```python
from build123d import *

# Parameters (mm, degrees)
ESQUISSE1_W             = 70
ESQUISSE1_H             = 55
ESQUISSE1_W_2           = 10
BOSS_EXTRU_1_DEPTH      = 2
ESQUISSE2_R             = 3.5
BOSS_EXTRU_2_DEPTH      = 6
ESQUISSE3_R             = 1.45
ENL_V_MAT_EXTRU_1_DEPTH = 4
ESQUISSE9_W             = 10
ESQUISSE9_H             = 55
BOSS_EXTRU_3_DEPTH      = 2
ESQUISSE10_R            = 6
ENL_V_MAT_EXTRU_8_DEPTH = 2
CONG_2_R                = 5
BOSS_EXTRU_4_DEPTH      = 5
BOSS_EXTRU_5_DEPTH      = 2
ESQUISSE15_R            = 2.15
BOSS_EXTRU_7_DEPTH      = 5
ESQUISSE17_W            = 8
ESQUISSE17_H            = 3
ENL_V_MAT_EXTRU_9_DEPTH = 10
CONG_3_R                = 1


with BuildPart() as part:
    # Esquisse1 → Boss.-Extru.1 (new body)
    with BuildSketch(Plane(origin=(0, 0, 0), x_dir=(1, 0, 0), z_dir=(0, 1, 0))):
        Rectangle(ESQUISSE1_W, ESQUISSE1_H)
        with Locations((-40, 0)):
            Rectangle(ESQUISSE1_W_2, ESQUISSE1_H)
    extrude(amount=BOSS_EXTRU_1_DEPTH)

    # Esquisse2 → Boss.-Extru.2 (add)
    with BuildSketch(Plane(origin=(0, 2, 0), x_dir=(1, 0, 0), z_dir=(0, 1, 0))):
        with Locations(Location((-11, 17.5, 0), (0, 0, 270))):
            Circle(ESQUISSE2_R)
        with Locations(Location((24, 17.5, 0), (0, 0, 270))):
            Circle(ESQUISSE2_R)
        with Locations(Location((24, -17.5, 0), (0, 0, 270))):
            Circle(ESQUISSE2_R)
        with Locations(Location((-11, -17.5, 0), (0, 0, 270))):
            Circle(ESQUISSE2_R)
    extrude(amount=BOSS_EXTRU_2_DEPTH)

    # Esquisse3 → Enlèv. mat.-Extru.1 (cut)
    with BuildSketch(Plane(origin=(0, 8, 0), x_dir=(1, 0, 0), z_dir=(0, 1, 0))):
        with Locations(Location((-11, 17.5, 0), (0, 0, 270))):
            Circle(ESQUISSE3_R)
        with Locations(Location((24, 17.5, 0), (0, 0, 270))):
            Circle(ESQUISSE3_R)
        with Locations(Location((24, -17.5, 0), (0, 0, 270))):
            Circle(ESQUISSE3_R)
        with Locations(Location((-11, -17.5, 0), (0, 0, 270))):
            Circle(ESQUISSE3_R)
    extrude(amount=-ENL_V_MAT_EXTRU_1_DEPTH, mode=Mode.SUBTRACT)

    # Esquisse9 → Boss.-Extru.3 (add)
    with BuildSketch(Plane(origin=(0, 2, 0), x_dir=(1, 0, 0), z_dir=(0, 1, 0))):
        with Locations((40, 0)):
            Rectangle(ESQUISSE9_W, ESQUISSE9_H)
    extrude(amount=-BOSS_EXTRU_3_DEPTH)

    # Esquisse10 → Enlèv. mat.-Extru.8 (cut)
    with BuildSketch(Plane(origin=(0, 2, 0), x_dir=(1, 0, 0), z_dir=(0, 1, 0))):
        with Locations(Location((35, 0, 0), (0, 0, 270))):
            Circle(ESQUISSE10_R)
    extrude(amount=-ENL_V_MAT_EXTRU_8_DEPTH, mode=Mode.SUBTRACT)

    # Congé2
    cong_2_edges = [part.edges().sort_by_distance(p)[0] for p in [
        (45, 1, -27.5),
        (45, 1, 27.5),
        (-45, 1, 27.5),
        (-45, 1, -27.5),
    ]]
    fillet(cong_2_edges, radius=CONG_2_R)

    # Esquisse12 → Boss.-Extru.4 (add)
    with BuildSketch(Plane(origin=(0, 2, 0), x_dir=(1, 0, 0), z_dir=(0, 1, 0))):
        with BuildLine():
            Line((40, 27.5), (-40, 27.5))
            ThreePointArc((-40, 27.5), (-43.535533906, 26.035533906), (-45, 22.5))
            Line((-45, 22.5), (-45, -22.5))
            ThreePointArc((-45, -22.5), (-43.535533906, -26.035533906), (-40, -27.5))
            Line((-40, -27.5), (40, -27.5))
            ThreePointArc((40, -27.5), (43.535533906, -26.035533906), (45, -22.5))
            Line((45, -22.5), (45, 22.5))
            ThreePointArc((45, 22.5), (43.535533906, 26.035533906), (40, 27.5))
        make_face()
        with BuildLine():
            Line((43, -22.5), (43, 22.5))
            ThreePointArc((43, 22.5), (42.121320344, 24.621320344), (40, 25.5))
            Line((40, 25.5), (-40, 25.5))
            ThreePointArc((-40, 25.5), (-42.121320344, 24.621320344), (-43, 22.5))
            Line((-43, 22.5), (-43, -22.5))
            ThreePointArc((-43, -22.5), (-42.121320344, -24.621320344), (-40, -25.5))
            Line((-40, -25.5), (40, -25.5))
            ThreePointArc((40, -25.5), (42.121320344, -24.621320344), (43, -22.5))
        make_face(mode=Mode.SUBTRACT)
    extrude(amount=BOSS_EXTRU_4_DEPTH)

    # Esquisse13 → Boss.-Extru.5 (add)
    with BuildSketch(Plane(origin=(0, 7, 0), x_dir=(1, 0, 0), z_dir=(0, 1, 0))):
        with BuildLine():
            Line((40, 27.5), (-40, 27.5))
            ThreePointArc((-40, 27.5), (-43.535533906, 26.035533906), (-45, 22.5))
            Line((-45, 22.5), (-45, -22.5))
            ThreePointArc((-45, -22.5), (-43.535533906, -26.035533906), (-40, -27.5))
            Line((-40, -27.5), (40, -27.5))
            ThreePointArc((40, -27.5), (43.535533906, -26.035533906), (45, -22.5))
            Line((45, -22.5), (45, 22.5))
            ThreePointArc((45, 22.5), (43.535533906, 26.035533906), (40, 27.5))
        make_face()
        with BuildLine():
            Line((40, 26.5), (-40, 26.5))
            ThreePointArc((-40, 26.5), (-42.828427125, 25.328427125), (-44, 22.5))
            Line((-44, 22.5), (-44, -22.5))
            ThreePointArc((-44, -22.5), (-42.828427125, -25.328427125), (-40, -26.5))
            Line((-40, -26.5), (40, -26.5))
            ThreePointArc((40, -26.5), (42.828427125, -25.328427125), (44, -22.5))
            Line((44, -22.5), (44, 22.5))
            ThreePointArc((44, 22.5), (42.828427125, 25.328427125), (40, 26.5))
        make_face(mode=Mode.SUBTRACT)
    extrude(amount=BOSS_EXTRU_5_DEPTH)

    # Esquisse15 → Boss.-Extru.7 (add)
    # profile 1 of 4: a face of its own
    with BuildSketch(Plane(origin=(0, 2, 0), x_dir=(1, 0, 0), z_dir=(0, 1, 0))):
        with BuildLine():
            ThreePointArc((-40, 17.35), (-36.358400077, 18.858400077), (-34.85, 22.5))
            Line((-34.85, 22.5), (-34.85, 25.5))
            Line((-34.85, 25.5), (-40, 25.5))
            ThreePointArc((-40, 25.5), (-42.121320344, 24.621320344), (-43, 22.5))
            Line((-43, 22.5), (-43, 17.35))
            Line((-43, 17.35), (-40, 17.35))
        make_face()
        with Locations(Location((-40, 22.5, 0), (0, 0, 270))):
            Circle(ESQUISSE15_R, mode=Mode.SUBTRACT)
    # profile 2 of 4: a face of its own
    with BuildSketch(Plane(origin=(0, 2, 0), x_dir=(1, 0, 0), z_dir=(0, 1, 0))):
        with BuildLine():
            Line((40, 25.5), (34.85, 25.5))
            Line((34.85, 25.5), (34.85, 22.5))
            ThreePointArc((34.85, 22.5), (36.358400077, 18.858400077), (40, 17.35))
            Line((40, 17.35), (43, 17.35))
            Line((43, 17.35), (43, 22.5))
            ThreePointArc((43, 22.5), (42.121320344, 24.621320344), (40, 25.5))
        make_face()
        with Locations(Location((40, 22.5, 0), (0, 0, 270))):
            Circle(ESQUISSE15_R, mode=Mode.SUBTRACT)
    # profile 3 of 4: a face of its own
    with BuildSketch(Plane(origin=(0, 2, 0), x_dir=(1, 0, 0), z_dir=(0, 1, 0))):
        with BuildLine():
            Line((43, -22.5), (43, -17.35))
            Line((43, -17.35), (40, -17.35))
            ThreePointArc((40, -17.35), (36.358400077, -18.858400077), (34.85, -22.5))
            Line((34.85, -22.5), (34.85, -25.5))
            Line((34.85, -25.5), (40, -25.5))
            ThreePointArc((40, -25.5), (42.121320344, -24.621320344), (43, -22.5))
        make_face()
        with Locations(Location((40, -22.5, 0), (0, 0, 270))):
            Circle(ESQUISSE15_R, mode=Mode.SUBTRACT)
    # profile 4 of 4: a face of its own
    with BuildSketch(Plane(origin=(0, 2, 0), x_dir=(1, 0, 0), z_dir=(0, 1, 0))):
        with BuildLine():
            Line((-40, -17.35), (-43, -17.35))
            Line((-43, -17.35), (-43, -22.5))
            ThreePointArc((-43, -22.5), (-42.121320344, -24.621320344), (-40, -25.5))
            Line((-40, -25.5), (-34.85, -25.5))
            Line((-34.85, -25.5), (-34.85, -22.5))
            ThreePointArc((-34.85, -22.5), (-36.358400077, -18.858400077), (-40, -17.35))
        make_face()
        with Locations(Location((-40, -22.5, 0), (0, 0, 270))):
            Circle(ESQUISSE15_R, mode=Mode.SUBTRACT)
    extrude(amount=BOSS_EXTRU_7_DEPTH)

    # Esquisse17 → Enlèv. mat.-Extru.9 (cut)
    with BuildSketch(Plane.ZY.offset(45)):
        with Locations((0, 4.5)):
            Rectangle(ESQUISSE17_W, ESQUISSE17_H)
    extrude(amount=-ENL_V_MAT_EXTRU_9_DEPTH, mode=Mode.SUBTRACT)

    # Congé3
    cong_3_edges = [part.edges().sort_by_distance(p)[0] for p in [
        (-44, 6, 4),
        (-44, 3, 4),
        (-44, 3, -4),
        (-44, 6, -4),
    ]]
    fillet(cong_3_edges, radius=CONG_3_R)


solid = part.part
```
Here's how the part is built. I have some questions about the finished solid (model axes, mm). Coordinates: 2 decimals unless noted, no trailing zeros. Order: outer loops, then holes, each group sorted by start corner. A loop starts at its lowest first (then second) coordinate and runs counter-clockwise, first axis right, second up.
1) Imagine slicing it at C-C on z = 8. List the corners of the cut face in (x, y) for me.
2) Will these pins go through, and if not, where does the flat tip stop? pin 1 (7 mm diameter, centred on x = 40, z = 22.5, fed in from -Y); pin 2 (12 mm diameter, centred on x = -24, z = 10, fed in from +Y); pin 3 (4.5 mm diameter, centred on x = 40.5, z = 23.5, fed in from +Y); pin 4 (1.5 mm diameter, centred on x = 41.5, y = 5, fed in from +Z).
3) I need wall thicknesses on line 1 (X direction, y = 3.5, z = 4.5); line 2 (Z direction, x = 34.5, y = 2.25); line 3 (Z direction, x = 21.5, y = 6). Which ranges of each line are inside material? Lowest first, please.
4) Imagine slicing it at A-A on z = 0. List the corners of the cut face in (x, y) for me, and give its area (3 significant figures).
5) We'd pull the mould along X, two halves only. Please class faces 1 (the face through (36.4, 4.46, 18.82)), 2 (the face through (-45, 6.4, -0.3)): +X half, -X half, draft (parallel to the pull), parting line (faces both ways), or undercut.
6) Imagine slicing it at B-B on x = -11. List the corners of the cut face in (y, z) for me.
Response values:
1. outline: (-45, 0) - (45, 0) - (45, 9) - (44, 9) - (44, 7) - (43, 7) - (43, 2) - (-43, 2) - (-43, 7) - (-44, 7) - (-44, 9) - (-45, 9) - close
2. pin 1: stops at y = 0
2. pin 2: stops at y = 2
2. pin 3: stops at y = 7
2. pin 4: stops at z = 27.44
3. line 1: x = -45 to -43, 43 to 45
3. line 2: z = -27.5 to -25.5, 25.5 to 27.5
3. line 3: z = -27.5 to -25.5, -19.95 to -15.05, 15.05 to 19.95, 25.5 to 27.5
4. outline: (-45, 0) - (29, 0) - (29, 2) - (-43, 2) - (-43, 3) - (-45, 3) - close; (-45, 6) - (-43, 6) - (-43, 7) - (-44, 7) - (-44, 9) - (-45, 9) - close; (41, 0) - (45, 0) - (45, 9) - (44, 9) - (44, 7) - (43, 7) - (43, 2) - (41, 2) - close
4. area: 174 mm2
5. face 1: undercut
5. face 2: -X half
6. outline: (0, -27.5) - (9, -27.5) - (9, -26.5) - (7, -26.5) - (7, -25.5) - (2, -25.5) - (2, -21) - (8, -21) - (8, -18.95) - (4, -18.95) - (4, -16.05) - (8, -16.05) - (8, -14) - (2, -14) - (2, 14) - (8, 14) - (8, 16.05) - (4, 16.05) - (4, 18.95) - (8, 18.95) - (8, 21) - (2, 21) - (2, 25.5) - (7, 25.5) - (7, 26.5) - (9, 26.5) - (9, 27.5) - (0, 27.5) - close
